Build history of the part. All positions in model axes, mm. Face numbers are marked on the shaded views. Give positions to 0.01 mm unless a question says otherwise; leave off trailing zeros. Write each loop counter-clockwise with the first axis right and the second up, starting at its lowest first coordinate (ties: lowest second). Pieces come first, ordered by that corner, then holes. Notation, with made-up numbers: (85.5, 75) -> (136.5, 75) arc R26 ccw to (136.5, 109) -> close; hole circle Ø5 at (8, -31.75). An arc over 180 degrees is marked (long way). Put each result on its own line as item: value.
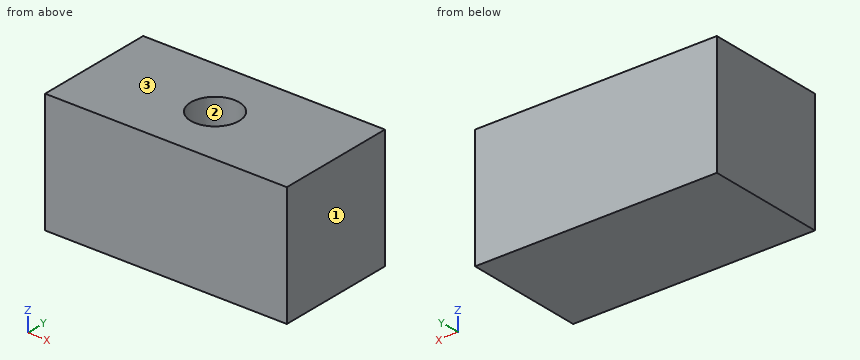
from build123d import *

# Parameters (mm, degrees)
SKETCH1_W           = 40
SKETCH1_H           = 20
BOSS_EXTRUDE1_DEPTH = 10
SKETCH2_R           = 4
CUT_EXTRUDE1_DEPTH  = 46.82575695


with BuildPart() as part:
    # Sketch1 → Boss-Extrude1 (new, symmetric)
    with BuildSketch(Plane.XY):
        with Locations((20, 10)):
            Rectangle(SKETCH1_W, SKETCH1_H)
    extrude(amount=BOSS_EXTRUDE1_DEPTH, both=True)

    # Sketch2 → Cut-Extrude1 (cut, through all)
    with BuildSketch(Plane.XY):
        with Locations((20, 10)):
            Circle(SKETCH2_R)
    extrude(amount=CUT_EXTRUDE1_DEPTH, mode=Mode.SUBTRACT)


solid = part.part
1) Pull direction X, two halves, no side cores. Call the marked faces 1, 2 and 3: released by +X, released by -X, zero draft, split by the parting line, or undercut.
Filled sheet:
face 1: released by +X
face 2: undercut
face 3: zero draft
2) Slice it at A-A (z = 5). Write the cut outline in (x, y).
Filled sheet:
outline: (0, 0) -> (40, 0) -> (40, 20) -> (0, 20) -> close; hole circle Ø8 at (20, 10)
3) Slice it at B-B (x = 20). Write the cut outline in (y, z), plus the area to 3 significant figures.
Filled sheet:
outline: (0, -10) -> (20, -10) -> (20, 10) -> (14, 10) -> (14, 0) -> (6, 0) -> (6, 10) -> (0, 10) -> close
area: 320 mm2
4) Wall check: L1, parallel to X at y = 10, z = 7; L2, parallel to Y at x = 20, z = 5; L3, parallel to Z at x = 19.5, y = 6.75. Give the ranges that are in metal, low to high.
Filled sheet:
L1: 0 to 16, 24 to 40
L2: 0 to 6, 14 to 20
L3: -10 to 0
5) Slice it at C-C (y = 10). Write the cut outline in (x, z).
Filled sheet:
outline: (0, -10) -> (40, -10) -> (40, 10) -> (24, 10) -> (24, 0) -> (16, 0) -> (16, 10) -> (0, 10) -> close
